For this review, take the finished solid that the model builds, in its own axes (mm). Give positions to 0.01 mm unless a question says otherwise; leave off trailing zeros. Loops run counter-clockwise (first coordinate to the right, second up) from the corner with the lowest first, then second, coordinate; pieces in that order, holes last. Notation, with made-up numbers: (3, -26.75) -> (33, -26.75) arc R15 cw to (33, -1.75) -> close; hole circle Ø10 at (-31.5, 43.5). An arc over 180 degrees is marked (long way). Answer as CSV lines item,"result". Start each with the question number.
Item 1: Clearance check with flat-ended pins moving along their axes: P1, Ø0.5, axis at y = 0.5, z = -8.5, coming from the -X side; P2, Ø0.5, axis at y = 0.5, z = -41, coming from the +X side; P3, Ø0.5, axis at y = 0.5, z = -54.5, coming from the -X side. State where each tip first meets the part, or that it passes through.
Item 2: For L1, parallel to X at y = 1.5, z = -48; L2, parallel to Z at x = 14.5, y = 0.7; L3, parallel to Z at x = 9.5, y = 1.2, list the stretches that pass through material, from the lowest coordinate up. Write a range as from..to.
Item 3: Add section A-A on z = -21. State the section outline as (x, y) points, plus the area to 3 significant figures.
Item 4: Add section B-B on x = 14.5. State the section outline as (y, z) points.
```python
from build123d import *

# Parameters (mm, degrees)
BOSS_EXTRUDE1_DEPTH = 1.8
FILLET2_R           = 0.5
SKETCH3_R           = 2.5
SKETCH3_R_2         = 1.75
BOSS_EXTRUDE2_DEPTH = 1.8
FILLET3_R           = 1


with BuildPart() as part:
    # Sketch1 → Boss-Extrude1 (new body)
    with BuildSketch(Plane(origin=(0, 0, 0), x_dir=(1, 0, 0), z_dir=(0, 1, 0))):
        with BuildLine():
            Line((0, 4.5), (0, 6.5))
            Line((0, 6.5), (6.1, 6.5))
            Line((6.1, 6.5), (6.1, 10.5))
            Line((6.1, 10.5), (10, 14.4))
            Line((10, 14.4), (10, 83.5))
            Line((10, 83.5), (16.4, 83.5))
            ThreePointArc((16.4, 83.5), (17.2719581, 81.425344658), (17.601960582, 79.199226044))
            Line((17.601960582, 79.199226044), (18.25, 49.5))
            Line((18.25, 49.5), (12, 49.5))
            Line((12, 49.5), (12, 37.18))
            add(Edge.make_bspline(
                [(12.5, 32.33), (12.5, 33.972282338), (12, 35.554764974), (12, 37.18)],
                knots=[0, 0, 0, 0, 1, 1, 1, 1], degree=3))
            Line((12.5, 32.33), (12.5, 3.07))
            ThreePointArc((12.5, 3.07), (11.600817818, 0.899182182), (9.43, 0))
            ThreePointArc((9.43, 0), (4.205660329, 1.182650422), (0, 4.5))
        make_face()
    extrude(amount=BOSS_EXTRUDE1_DEPTH)

    # Fillet2
    fillet2_edges = [part.edges().sort_by_distance(p)[0] for p in [
        (0, 0.9, -6.5),
        (6.1, 0.9, -6.5),
        (6.1, 0.9, -10.5),
        (10, 0.9, -14.4),
        (10, 0.9, -83.5),
        (18.25, 0.9, -49.5),
        (12, 0.9, -49.5),
    ]]
    fillet(fillet2_edges, radius=FILLET2_R)

    # Sketch3 → Boss-Extrude2 (add)
    with BuildSketch(Plane.XZ):
        with Locations((9.5, 2.499832541)):
            Circle(SKETCH3_R)
        with Locations((9.5, 2.499832541)):
            Circle(SKETCH3_R_2, mode=Mode.SUBTRACT)
        with BuildLine():
            ThreePointArc((11.824045318, 1.578521867), (9.031018815, 0.044215175), (7, 2.499832541))
            Line((7, 2.499832541), (7, -0.245881701))
            ThreePointArc((7, -0.245881701), (8.2087959, -0.061626967), (9.43, 0))
            ThreePointArc((9.43, 0), (10.256451345, -0.113333266), (11.021883517, -0.444965358))
            Line((11.021883517, -0.444965358), (11.824045318, 1.578521867))
        make_face()
        with BuildLine():
            ThreePointArc((9.43, 0), (8.2087959, -0.061626967), (7, -0.245881701))
            Line((7, -0.245881701), (7, -0.500167459))
            Line((7, -0.500167459), (11, -0.500167459))
            Line((11, -0.500167459), (11.021883517, -0.444965358))
            ThreePointArc((11.021883517, -0.444965358), (10.256451345, -0.113333266), (9.43, 0))
        make_face()
    extrude(amount=-BOSS_EXTRUDE2_DEPTH)

    # Fillet3
    fillet3_edges = [part.edges().sort_by_distance(p)[0] for p in [
        (7, 0.9, -0.245881701),
        (11.021883517, 0.9, -0.444965358),
    ]]
    fillet(fillet3_edges, radius=FILLET3_R)


solid = part.part
```
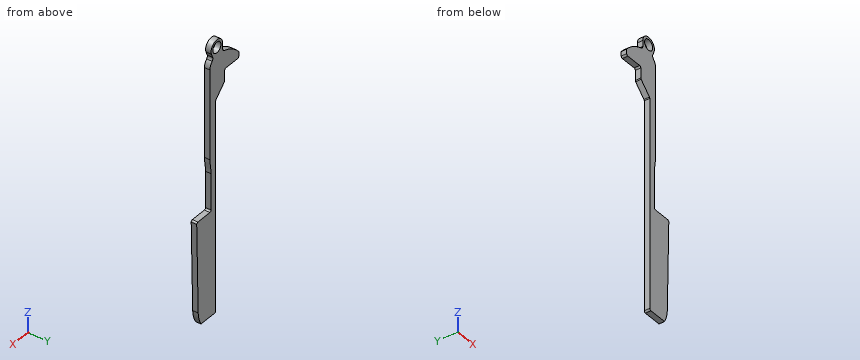
Computed values:
1,P1,"x = 6.1"
1,P2,"x = 12"
1,P3,"x = 10"
2,L1,"10..12"
2,L2,"-83.5..-49.5"
2,L3,"-13.9..0.75, 4.25..5"
3,outline,"(10, 0) -> (12.5, 0) -> (12.5, 1.8) -> (10, 1.8) -> close"
3,area,"4.50 mm²"
4,outline,"(0, -83.5) -> (1.8, -83.5) -> (1.8, -49.5) -> (0, -49.5) -> close"
